```python
from build123d import *

# Parameters (mm, degrees)
SKETCH1_W           = 11.89
SKETCH1_H           = 20
BOSS_EXTRUDE1_DEPTH = 79
SKETCH4_R           = 2.15
CUT_EXTRUDE1_DEPTH  = 6.82
SKETCH5_R           = 2.15
CUT_EXTRUDE2_DEPTH  = 6.825


with BuildPart() as part:
    # Sketch1 → Boss-Extrude1 (new body)
    with BuildSketch(Plane.XY):
        with Locations((5.945, 10)):
            Rectangle(SKETCH1_W, SKETCH1_H)
    extrude(amount=BOSS_EXTRUDE1_DEPTH)

    # Sketch4 → Cut-Extrude1 (cut)
    with BuildSketch(Plane.ZY):
        with Locations((39.5, 10)):
            Circle(SKETCH4_R)
        with Locations((9.5, 10)):
            Circle(SKETCH4_R)
        with Locations((69.5, 10)):
            Circle(SKETCH4_R)
    extrude(amount=-CUT_EXTRUDE1_DEPTH, mode=Mode.SUBTRACT)

    # Sketch5 → Cut-Extrude2 (cut)
    with BuildSketch(Plane.XZ):
        with Locations((5.945, 39.5)):
            Circle(SKETCH5_R)
        with Locations((5.945, 69.5)):
            Circle(SKETCH5_R)
        with Locations((5.945, 9.5)):
            Circle(SKETCH5_R)
    extrude(amount=-CUT_EXTRUDE2_DEPTH, mode=Mode.SUBTRACT)


solid = part.part
```
The model under review builds one solid part; all positions refer to its coordinate system, in mm. A direction names the side the tool comes from. Give positions to 0.01 mm unless a question says otherwise; leave off trailing zeros. Write each loop counter-clockwise with the first axis right and the second up, starting at its lowest first coordinate (ties: lowest second). Pieces come first, ordered by that corner, then holes. Notation, with made-up numbers: M -32.5,89.5 L -5.5,89.5 A24 ccw -5.5,102.5 Z; hole C -10,-27.75 d2. An arc over 180 degrees is marked long. Write each question's results on one line, items separated by ' | '. Start each with the question number.
1. Mouldability with a two-part tool opening along X and no side actions: class faces 1 (the cylindrical face through (5.665, 3.365, 41.632)), 2 (the flat face through (11.89, 10, 39)), 3 (the flat face through (6.82, 10, 69)), 4 (the flat face through (6, 10, 0)) as released by +X, released by -X, zero draft, split by the parting line, or undercut.
2. We need section B-B (x = 2.5). Write out the cut boundary in (y, z), and give its area (3 significant figures).
3. For probe 1 along Z at (x, y) = (4.5, 10.25); probe 2 along Y at (x, z) = (2.75, 69.5); probe 3 along Z at (x, y) = (6, 8.5), list the stretches that pass through material, from the lowest coordinate up. Write a range as [from, to].
4. We need section C-C (y = 10). Write out the cut boundary in (x, z).
5. Insertion check: pin 1 Ø3 at (x, y) = (5, 15) entering from -Z; pin 2 Ø4 at (y, z) = (10, 9.5) entering from -X; pin 3 Ø2 at (x, z) = (5.5, 10.5) entering from -Y (3 decimals). Each pin has a flat end and moves straight along its axis. Give the tip position at first contact, or say it passes through.
6. We need section D-D (z = 69.5). Write out the cut boundary in (x, y) (3 decimals), and give its area (3 significant figures).
7. We need section A-A (y = 1.5). Write out the cut boundary in (x, z) (3 decimals), and give its area (3 significant figures).
8. For faces 5 (the flat face through (9, 0, 39)), 6 (the flat face through (6, 6.825, 70)), 7 (the flat face through (6.82, 10, 39)), list the 3-axis set-ups (+Z, -Z, +X, -X, +Y, -Y) from which the entire face can be reached by the end or side of a thin tool; tool diameter is ignored.
Results found:
1) face 1: undercut | face 2: released by +X | face 3: released by -X | face 4: zero draft
2) outline: M 0,0 L 20,0 L 20,79 L 0,79 Z; hole C 10,9.5 d4.3; hole C 10,39.5 d4.3; hole C 10,69.5 d4.3 | area: 1,540 mm^2
3) probe 1: z = [0, 7.36], [11.64, 37.36], [41.64, 67.36], [71.64, 79] | probe 2: y = [0, 7.85], [12.15, 20] | probe 3: z = [0, 7.96], [11.04, 37.96], [41.04, 67.96], [71.04, 79]
4) outline: M 0,0 L 11.89,0 L 11.89,79 L 0,79 L 0,71.65 L 6.82,71.65 L 6.82,67.35 L 0,67.35 L 0,41.65 L 6.82,41.65 L 6.82,37.35 L 0,37.35 L 0,11.65 L 6.82,11.65 L 6.82,7.35 L 0,7.35 Z
5) pin 1: stops at z = 0 | pin 2: stops at x = 6.82 | pin 3: stops at y = 6.825
6) outline: M 0,0 L 3.795,0 L 3.795,6.825 L 8.095,6.825 L 8.095,0 L 11.89,0 L 11.89,20 L 0,20 L 0,12.15 L 6.82,12.15 L 6.82,7.85 L 0,7.85 Z | area: 179 mm^2
7) outline: M 0,0 L 11.89,0 L 11.89,79 L 0,79 Z; hole C 5.945,9.5 d4.3; hole C 5.945,39.5 d4.3; hole C 5.945,69.5 d4.3 | area: 896 mm^2
8) face 5: +Z, -Z, +X, -X, -Y | face 6: -Y | face 7: -X
